```python
from build123d import *

# Parameters (mm, degrees)
SKETCH_2_W          = 170
SKETCH_2_H          = 20
EXTRUDE_1_DEPTH     = 23
CUT_EXTRUDE_1_DEPTH = 173.710740836
SKETCH_4_W          = 17
SKETCH_4_H          = 13
CUT_EXTRUDE_2_DEPTH = 30
CUT_EXTRUDE_3_DEPTH = 173.710740836
SKETCH_6_W          = 87.5
SKETCH_6_H          = 63
EXTRUDE_2_DEPTH     = 3
SKETCH_7_R          = 1.25
CUT_EXTRUDE_4_DEPTH = 186.632028486
SKETCH_7_3_R        = 2
CUT_EXTRUDE_5_DEPTH = 1.5
CUT_EXTRUDE_6_DEPTH = 186.632028486
FILLET_2_R          = 4
SKETCH_10_R         = 0.9
CUT_EXTRUDE_7_DEPTH = 186.178967488
SKETCH_9_W          = 78.5
SKETCH_9_H          = 16.208535094
CUT_EXTRUDE_8_DEPTH = 191.475720238


with BuildPart() as part:
    # 草图2 → 凸台-拉伸1 (new body)
    with BuildSketch(Plane(origin=(0, 0, 0), x_dir=(1, 0, 0), z_dir=(0, 1, 0))):
        with Locations((85, -10)):
            Rectangle(SKETCH_2_W, SKETCH_2_H)
    extrude(amount=EXTRUDE_1_DEPTH)

    # 草图3 → 切除-拉伸1 (cut, through all)
    with BuildSketch(Plane(origin=(0, 23, 0), x_dir=(1, 0, 0), z_dir=(0, 1, 0))):
        with BuildLine():
            ThreePointArc((161.6, -10), (159.341699476, -8.541699476), (158.941699476, -11.2))
            Line((158.941699476, -11.2), (161.058300524, -11.2))
            ThreePointArc((161.058300524, -11.2), (161.458300524, -10.658300524), (161.6, -10))
        make_face()
        with BuildLine():
            ThreePointArc((126.6, -10), (124.341699476, -8.541699476), (123.941699476, -11.2))
            Line((123.941699476, -11.2), (126.058300524, -11.2))
            ThreePointArc((126.058300524, -11.2), (126.458300524, -10.658300524), (126.6, -10))
        make_face()
    extrude(amount=-CUT_EXTRUDE_1_DEPTH, mode=Mode.SUBTRACT)

    # 草图4 → 切除-拉伸2 (cut)
    with BuildSketch(Plane(origin=(170, 0, 0), x_dir=(0, 0, -1), z_dir=(1, 0, 0))):
        with Locations((-8.5, 11.5)):
            Rectangle(SKETCH_4_W, SKETCH_4_H)
    extrude(amount=-CUT_EXTRUDE_2_DEPTH, mode=Mode.SUBTRACT)

    # 草图5 → 切除-拉伸3 (cut, through all)
    with BuildSketch(Plane(origin=(0, 23, 0), x_dir=(1, 0, 0), z_dir=(0, 1, 0))):
        with BuildLine():
            Line((117.5, -17), (117.5, -10))
            ThreePointArc((117.5, -10), (125, -2.5), (132.5, -10))
            Line((132.5, -10), (132.5, -17))
            Line((132.5, -17), (152.5, -17))
            Line((152.5, -17), (152.5, -10))
            ThreePointArc((152.5, -10), (160, -2.5), (167.5, -10))
            Line((167.5, -10), (167.5, -17))
            Line((167.5, -17), (170, -17))
            Line((170, -17), (170, 0))
            Line((170, 0), (0, 0))
            Line((0, 0), (0, -20))
            Line((0, -20), (102.5, -20))
            Line((102.5, -20), (102.5, -17))
            Line((102.5, -17), (117.5, -17))
        make_face()
    extrude(amount=-CUT_EXTRUDE_3_DEPTH, mode=Mode.SUBTRACT)

    # 草图6 → 凸台-拉伸2 (add)
    with BuildSketch(Plane.XY.offset(20)):
        with Locations((136.25, 11.5)):
            Rectangle(SKETCH_6_W, SKETCH_6_H)
    extrude(amount=-EXTRUDE_2_DEPTH)

    # 草图7 → 切除-拉伸4 (cut, through all)
    with BuildSketch(Plane(origin=(0, 0, 17), x_dir=(-1, 0, 0), z_dir=(0, 0, -1))):
        with Locations((-174, 35)):
            Circle(SKETCH_7_R)
        with Locations((-107.5, 35)):
            Circle(SKETCH_7_R)
        with Locations((-107.5, -12)):
            Circle(SKETCH_7_R)
        with Locations((-174, -12)):
            Circle(SKETCH_7_R)
    extrude(amount=-CUT_EXTRUDE_4_DEPTH, mode=Mode.SUBTRACT)

    # 草图7<3> → 切除-拉伸5 (cut)
    with BuildSketch(Plane(origin=(0, 0, 17), x_dir=(-1, 0, 0), z_dir=(0, 0, -1))):
        with Locations((-174, 35)):
            Circle(SKETCH_7_3_R)
        with Locations((-107.5, 35)):
            Circle(SKETCH_7_3_R)
        with Locations((-174, -12)):
            Circle(SKETCH_7_3_R)
        with Locations((-107.5, -12)):
            Circle(SKETCH_7_3_R)
    extrude(amount=-CUT_EXTRUDE_5_DEPTH, mode=Mode.SUBTRACT)

    # 草图8 → 切除-拉伸6 (cut, through all)
    with BuildSketch(Plane(origin=(0, 0, 17), x_dir=(-1, 0, 0), z_dir=(0, 0, -1))):
        Polygon((-180, 43), (-180, 41), (-101.5, 41), (-101.5, -18), (-180, -18), (-180, -20), (-92.5, -20), (-92.5, 43), align=None)
    extrude(amount=-CUT_EXTRUDE_6_DEPTH, mode=Mode.SUBTRACT)

    # 圆角2
    fillet_2_edges = [part.edges().sort_by_distance(p)[0] for p in [
        (101.5, -18, 18.5),
        (101.5, 41, 18.5),
        (180, 41, 18.5),
        (180, -18, 18.5),
    ]]
    fillet(fillet_2_edges, radius=FILLET_2_R)

    # 草图10 → 切除-拉伸7 (cut, through all)
    with BuildSketch(Plane(origin=(0, 0, 17), x_dir=(-1, 0, 0), z_dir=(0, 0, -1))):
        with Locations((-170.5, 20.5)):
            Circle(SKETCH_10_R)
        with Locations((-149.5, 20.5)):
            Circle(SKETCH_10_R)
        with Locations((-170.5, 2.5)):
            Circle(SKETCH_10_R)
        with Locations((-149.5, 2.5)):
            Circle(SKETCH_10_R)
        with Locations((-135.5, 4)):
            Circle(SKETCH_10_R)
        with Locations((-135.5, 19)):
            Circle(SKETCH_10_R)
        with Locations((-114.5, 19)):
            Circle(SKETCH_10_R)
        with Locations((-114.5, 4)):
            Circle(SKETCH_10_R)
    extrude(amount=-CUT_EXTRUDE_7_DEPTH, mode=Mode.SUBTRACT)

    # 草图9 → 切除-拉伸8 (cut, through all)
    with BuildSketch(Plane.XZ.offset(18)):
        with Locations((140.75, 8.895732453)):
            Rectangle(SKETCH_9_W, SKETCH_9_H)
    extrude(amount=-CUT_EXTRUDE_8_DEPTH, mode=Mode.SUBTRACT)


solid = part.part
```
Input: part model. Units: mm. Frame: model coordinates. A direction names the side the tool comes from. Give positions to 0.01 mm unless a question says otherwise; leave off trailing zeros. Order: outer loops, then holes, each group sorted by start corner. A loop starts at its lowest first (then second) coordinate and runs counter-clockwise, first axis right, second up. Notation, with made-up numbers: (13, 26) - (19, 26) arc R31 cw to (19, 59) - close; hole circle Ø5 at (-22, 23). An arc over 180 degrees is marked (long way). One line per item, written item: value.
1. Line query: probe 1 along Y at (x, z) = (107.5, 17.95); probe 2 along Y at (x, z) = (135.5, 17.95); probe 3 along X at (y, z) = (-15, 17.35). Output: solid intervals per line, ascending.
Determined:
probe 1: -18 to -14, -10 to 33, 37 to 41
probe 2: -18 to 3.1, 4.9 to 18.1, 19.9 to 41
probe 3: 101.63 to 179.87
2. Cut plane C-C, the plane z = 17.5. Give the number of separate pieces and of enclosed holes in the cut face, and give its area (3 significant figures).
Determined:
separate pieces: 1
enclosed holes: 12
area: 4,550 mm2
3. Cut plane B-B, the plane y = -12. Output: boundary loops of the cut face in (x, z).
Determined:
outline: (101.5, 17) - (105.5, 17) - (105.5, 18.5) - (106.25, 18.5) - (106.25, 20) - (101.5, 20) - close; (108.75, 18.5) - (109.5, 18.5) - (109.5, 17) - (172, 17) - (172, 18.5) - (172.75, 18.5) - (172.75, 20) - (108.75, 20) - close; (175.25, 18.5) - (176, 18.5) - (176, 17) - (180, 17) - (180, 20) - (175.25, 20) - close
4. Reachability of faces 1 (the face through (176, -12, 18)), 2 (the face through (171.16, 21.11, 18.48)) from +Z, -Z, +X, -X, +Y, -Y: full face, straight path, thin tool, end or side. Return the list, or none.
Determined:
face 1: -Z
face 2: +Z, -Z
5. Pin query (flat end, axial travel): pin 1 Ø3 at (x, y) = (107.5, 35) entering from -Z; pin 2 Ø1.6 at (x, y) = (114.5, 4) entering from -Z. Return the tip coordinate at first contact, or that it passes through.
Determined:
pin 1: z = 18.5
pin 2: through
6. Cut plane A-A, the plane x = 174. Output: boundary loops of the cut face in (y, z), and give its area (4 significant figures).
Determined:
outline: (-18, 17) - (-14, 17) - (-14, 18.5) - (-13.25, 18.5) - (-13.25, 20) - (-18, 20) - close; (-10.75, 18.5) - (-10, 18.5) - (-10, 17) - (33, 17) - (33, 18.5) - (33.75, 18.5) - (33.75, 20) - (-10.75, 20) - close; (36.25, 18.5) - (37, 18.5) - (37, 17) - (41, 17) - (41, 20) - (36.25, 20) - close
area: 157.5 mm2
7. Draft query along X for faces 3 (the face through (180, 11, 19)), 4 (the face through (101.5, 12, 18)), 5 (the face through (150.16, 21.11, 18.48)), 6 (the face through (140, -18, 18)). Return one class per face: released by +X, released by -X, zero draft, split by the parting line, or undercut.
Determined:
face 3: released by +X
face 4: released by -X
face 5: undercut
face 6: zero draft
